```python
from build123d import *

# Parameters (mm, degrees)
MODEL_R             = 3
BOSS_EXTRUDE1_DEPTH = 6


with BuildPart() as part:
    # Model → Boss-Extrude1 (new body)
    with BuildSketch(Plane.XY):
        with BuildLine():
            Line((24.94501548, 21.95092931), (48.44501548, 21.95092931))
            ThreePointArc((48.44501548, 21.95092931), (56.44501548, 13.95092931), (48.44501548, 5.95092931))
            Line((48.44501548, 5.95092931), (24.94501548, 5.95092931))
            ThreePointArc((24.94501548, 5.95092931), (16.94501548, 13.95092931), (24.94501548, 21.95092931))
        make_face()
        with Locations((36.69501548, 13.993666272)):
            Circle(MODEL_R, mode=Mode.SUBTRACT)
        Polygon((27.69501548, 13.95092931), (27.69501548, 16.70092931), (22.19501548, 16.70092931), (22.19501548, 11.20092931), (27.69501548, 11.20092931), align=None, mode=Mode.SUBTRACT)
        Polygon((45.69501548, 13.95092931), (45.69501548, 16.70092931), (51.19501548, 16.70092931), (51.19501548, 11.20092931), (45.69501548, 11.20092931), align=None, mode=Mode.SUBTRACT)
    extrude(amount=BOSS_EXTRUDE1_DEPTH)


solid = part.part
```
Verification items for the finished model (mm, model axes). A direction names the side the tool comes from. Round coordinates to 2 decimals unless told otherwise and drop trailing zeros. Write each loop counter-clockwise with the first axis right and the second up, starting at its lowest first coordinate (ties: lowest second). Pieces come first, ordered by that corner, then holes. Notation, with made-up numbers: (-34, 23) - (-14, 23) arc R12 ccw to (-14, 39) - close; hole circle Ø1 at (73.25, -16). An arc over 180 degrees is marked (long way). Answer as a JSON object with one key per item and string values. Group by question number.
Q1. Thickness scan on line 1 (Y direction, x = 46.5, z = 4.05); line 2 (X direction, y = 13.5, z = 1.5); line 3 (X direction, y = 11.5, z = 4.8). Record the ranges inside material, lowest first.
Q2. Section check B-B, the plane y = 13.25. Enter the section's corners in (x, z).
Q3. Go/stop test with flat-tipped pins: pin 1 Ø1.6 at (y, z) = (15, 1.5) entering from +X; pin 2 Ø5.5 at (x, y) = (36.7, 13.99) entering from +Z. Record where each tip stops, or that it passes through.
Q4. Mould release check, pull along Y, two halves, no side actions. Record for faces 3 (the cylindrical face through (16.947, 13.775, 2.958)), 4 (the cylindrical face through (39.56, 14.89, 2.96)), 5 (the flat face through (37, 5.951, 3)): released by +Y, released by -Y, zero draft, split by the parting line, or undercut.
Q5. Tool access check on faces 1 (the flat face through (25, 16.701, 3)), 2 (the flat face through (37, 21.951, 3)). Record the directions out of +Z, -Z, +X, -X, +Y, -Y that give a thin tool (end or side, any length) a straight path to the whole face; none if there is none.
Q6. Section check C-C, the plane z = 0.55. Enter the section's corners in (x, y).
Q7. Section check A-A, the plane x = 47.5. Enter the section's corners in (y, z).
Q8. Section check D-D, the plane y = 19. Enter the section's corners in (x, z), plus the area to 3 significant figures.
Found:
{
 "1": {"line 1": "y = 5.95 to 11.2, 16.7 to 21.95", "line 2": "x = 16.96 to 22.2, 27.7 to 33.74, 39.65 to 45.7, 51.2 to 56.43", "line 3": "x = 17.33 to 22.2, 27.7 to 35.03, 38.36 to 45.7, 51.2 to 56.06"},
 "2": {"outline": "(16.98, 0) - (22.2, 0) - (22.2, 6) - (16.98, 6) - close; (27.7, 0) - (33.79, 0) - (33.79, 6) - (27.7, 6) - close; (39.6, 0) - (45.7, 0) - (45.7, 6) - (39.6, 6) - close; (51.2, 0) - (56.41, 0) - (56.41, 6) - (51.2, 6) - close"},
 "3": {"pin 1": "stops at x = 56.44", "pin 2": "passes through"},
 "4": {"face 3": "split by the parting line", "face 4": "undercut", "face 5": "released by -Y"},
 "5": {"face 1": "+Z, -Z", "face 2": "+Z, -Z, +X, -X, +Y"},
 "6": {"outline": "(24.95, 5.95) - (48.45, 5.95) arc R8 ccw to (48.45, 21.95) - (24.95, 21.95) arc R8 ccw to start; hole (22.2, 11.2) - (27.7, 11.2) - (27.7, 16.7) - (22.2, 16.7) - close; hole circle Ø6 at (36.7, 13.99); hole (45.7, 11.2) - (51.2, 11.2) - (51.2, 16.7) - (45.7, 16.7) - close"},
 "7": {"outline": "(5.95, 0) - (11.2, 0) - (11.2, 6) - (5.95, 6) - close; (16.7, 0) - (21.95, 0) - (21.95, 6) - (16.7, 6) - close"},
 "8": {"outline": "(18.74, 0) - (54.65, 0) - (54.65, 6) - (18.74, 6) - close", "area": "215 mm^2"}
}
